from build123d import *

# Parameters (mm, degrees)
PAD012_DEPTH    = 3
SKETCH047_R     = 1.45
POCKET013_DEPTH = 27
FILLET010_R     = 1.5
FILLET018_R     = 0.5


with BuildPart() as part:
    # Sketch036 → Pad012 (new body)
    with BuildSketch(Plane.XY):
        with BuildLine():
            add(Edge.make_bspline(
                [(132.333333, -29.811537), (140.031799, -32.510384), (146.350027, -35.078621), (153.231854, -38.154949)],
                knots=[0, 0, 0, 0, 1, 1, 1, 1], degree=3))
            Line((153.231854, -38.154949), (175.310198, 11.234895))
            add(Edge.make_bspline(
                [(150.875, 88.9625), (150.875, 42.8625), (150.875, 22.157965), (175.310198, 11.234895)],
                knots=[0, 0, 0, 0, 1, 1, 1, 1], degree=3))
            add(Edge.make_bspline(
                [(132.333333, 89.593483), (137.531693, 89.226463), (141.793335, 88.990242), (150.875, 88.9625)],
                knots=[0, 0, 0, 0, 1, 1, 1, 1], degree=3))
            Line((132.333333, 89.593483), (132.333333, -29.811537))
        make_face()
    extrude(amount=PAD012_DEPTH)

    # Sketch047 → Pocket013 (cut)
    with BuildSketch(Plane.XY):
        with Locations((-4.375, -4.375)):
            Circle(SKETCH047_R)
        with Locations((-4.375, 80.575)):
            Circle(SKETCH047_R)
        with Locations((151.401832, -33.366184)):
            Circle(SKETCH047_R)
        with Locations((170.521433, 9.404873)):
            Circle(SKETCH047_R)
        with Locations((147.25, 85.3375)):
            Circle(SKETCH047_R)
        with Locations((43.25, -13.9)):
            Circle(SKETCH047_R)
        with Locations((57.15, 92.085)):
            Circle(SKETCH047_R)
        with Locations((95.25, 92.085)):
            Circle(SKETCH047_R)
        with Locations((95.25, -13.9)):
            Circle(SKETCH047_R)
    extrude(amount=POCKET013_DEPTH, mode=Mode.SUBTRACT)

    # Fillet010
    fillet010_edges = [part.edges().sort_by_distance(p)[0] for p in [
        (175.310198, 11.234895, 1.5),
        (150.875, 88.9625, 1.5),
        (153.231854, -38.154949, 1.5),
    ]]
    fillet(fillet010_edges, radius=FILLET010_R)

    # Fillet018
    fillet018_edges = [part.edges().sort_by_distance(p)[0] for p in [
        (132.333333, 89.593483, 1.5),
        (132.333333, -29.811537, 1.5),
    ]]
    fillet(fillet018_edges, radius=FILLET018_R)


with BuildPart() as part_1:
    # Body011 placement: moved
    add(part.part.moved(Location((0, 0, -24))))


solid = part_1.part
Read the model definition and answer for the solid it produces. Units are mm, in the model's axes. Round coordinates to 2 decimals unless told otherwise and drop trailing zeros. Order: outer loops, then holes, each group sorted by start corner. A loop starts at its lowest first (then second) coordinate and runs counter-clockwise, first axis right, second up. Notation, with made-up numbers: (11, 74.5) - (21, 74.5) arc R13 ccw to (21, 98.5) - close; hole circle Ø2 at (13.25, -12.5). An arc over 180 degrees is marked (long way). Use one line per item in the form item = value. Start each with the question number.
(1) The part is cut by section B-B (z = -22.4). Count the separate pieces of the cut face and the enclosed holes in it, then the cut area to 3 significant figures.
(2) Find the intervals of material crossed by line 1 along X through (y, z) = (9.5, -23.05); line 2 along Y through (x, z) = (147.25, -21.95); line 3 along Y through (x, z) = (171, -21.3), in increasing order. Write a range as from..to.
(3) Determine the mould class of faces 1 (the face through (164.13, -13.78, -22.52)), 2 (the face through (150, -33, -23)), 3 (the face through (132.333, 31, -23)) for opening direction Y: +Y half, -Y half, draft (parallel to the pull), parting line (faces both ways), or undercut.
(4) Flat-ended cylindrical pins translate along their axes: pin 1 Ø3.5 at (x, y) = (151.4, -33.37) entering from +Z; pin 2 Ø1.5 at (x, z) = (168.5, -23.5) entering from -Y. Find the tip coordinate at first contact, or state that the pin passes through.
(5) The part is cut by section A-A (y = 5). Give the vertices of the cut face in (x, z).
Checked values:
q1.separate_pieces = 1
q1.enclosed_holes = 3
q1.area = 3,200 mm^2
q2.line_1 = 132.33..169.07, 171.97..174.53
q2.line_2 = -35.55..83.89, 86.79..88.99
q2.line_3 = 1.59..8.04, 10.77..13.41
q3.face_1 = -Y half
q3.face_2 = undercut
q3.face_3 = draft
q4.pin_1 = -21
q4.pin_2 = -5.68
q5.outline = (132.33, -24) - (172.52, -24) - (172.52, -21) - (132.33, -21) - close
